```python
from build123d import *

# Parameters (mm, degrees)
SKETCH_1_W          = 15
SKETCH_1_H          = 170
EXTRUDE_1_DEPTH     = 12
SKETCH_2_W          = 8.1
SKETCH_2_H          = 10.1
CUT_EXTRUDE_1_DEPTH = 20.5
CUT_EXTRUDE_2_REACH = 89.144
SKETCH_3_R          = 2.1
SKETCH_5_R          = 2.1
CUT_EXTRUDE_3_DEPTH = 12
SKETCH_6_W          = 15
SKETCH_6_H          = 12
CUT_EXTRUDE_4_DEPTH = 2


with BuildPart() as part:
    # 草图1 → 凸台-拉伸1 (new body)
    with BuildSketch(Plane.XY):
        Rectangle(SKETCH_1_W, SKETCH_1_H)
    extrude(amount=EXTRUDE_1_DEPTH)

    # 草图2 → 切除-拉伸1 (cut)
    with BuildSketch(Plane.XZ.offset(85)):
        with Locations((-1.5, 5.05)):
            Rectangle(SKETCH_2_W, SKETCH_2_H)
    extrude(amount=-CUT_EXTRUDE_1_DEPTH, mode=Mode.SUBTRACT)

    # 切除-拉伸2: up to this face of the body (flat: up to its plane)
    cut_extrude_2_end = Plane(part.part.faces().sort_by_distance((-7.5, 0, 6))[0])
    # 草图3 → 切除-拉伸2 (cut, up to the picked face)
    with BuildSketch(Plane(origin=(7.5, 0, 0), x_dir=(0, 0, -1), z_dir=(1, 0, 0)), mode=Mode.PRIVATE) as cut_extrude_2_sk1:
        with Locations((-5, -69.75)):
            Circle(SKETCH_3_R)
    cut_extrude_2_tool1 = split(extrude(cut_extrude_2_sk1.sketch, amount=-CUT_EXTRUDE_2_REACH, mode=Mode.PRIVATE), bisect_by=cut_extrude_2_end, keep=Keep.BOTH, mode=Mode.PRIVATE)
    # 草图3 → 切除-拉伸2 (cut, up to the picked face)
    with BuildSketch(Plane(origin=(7.5, 0, 0), x_dir=(0, 0, -1), z_dir=(1, 0, 0)), mode=Mode.PRIVATE) as cut_extrude_2_sk2:
        with Locations((-5, -78.75)):
            Circle(SKETCH_3_R)
    cut_extrude_2_tool2 = split(extrude(cut_extrude_2_sk2.sketch, amount=-CUT_EXTRUDE_2_REACH, mode=Mode.PRIVATE), bisect_by=cut_extrude_2_end, keep=Keep.BOTH, mode=Mode.PRIVATE)
    add(cut_extrude_2_tool1.solids().sort_by(Axis((7.5, -69.75, 5), (-1, 0, 0)))[0], mode=Mode.SUBTRACT)
    add(cut_extrude_2_tool2.solids().sort_by(Axis((7.5, -78.75, 5), (-1, 0, 0)))[0], mode=Mode.SUBTRACT)

    # 草图5 → 切除-拉伸3 (cut)
    with BuildSketch(Plane.XY.offset(12)):
        with Locations((0, -27)):
            Circle(SKETCH_5_R)
        with Locations((0, -35)):
            Circle(SKETCH_5_R)
        with Locations((0, -19)):
            Circle(SKETCH_5_R)
        with Locations((0, -11)):
            Circle(SKETCH_5_R)
        with Locations((0, -3)):
            Circle(SKETCH_5_R)
        with Locations((0, 5)):
            Circle(SKETCH_5_R)
        with Locations((0, 13)):
            Circle(SKETCH_5_R)
        with Locations((0, 21)):
            Circle(SKETCH_5_R)
        with Locations((0, 29)):
            Circle(SKETCH_5_R)
        with Locations((0, 37)):
            Circle(SKETCH_5_R)
        with Locations((0, 45)):
            Circle(SKETCH_5_R)
        with Locations((0, 53)):
            Circle(SKETCH_5_R)
        with Locations((0, 61)):
            Circle(SKETCH_5_R)
        with Locations((0, 69)):
            Circle(SKETCH_5_R)
    extrude(amount=-CUT_EXTRUDE_3_DEPTH, mode=Mode.SUBTRACT)

    # 草图6 → 切除-拉伸4 (cut)
    with BuildSketch(Plane.XZ.offset(85)):
        with Locations((0, 6)):
            Rectangle(SKETCH_6_W, SKETCH_6_H)
    extrude(amount=-CUT_EXTRUDE_4_DEPTH, mode=Mode.SUBTRACT)


solid = part.part
```
Input: part model. Units: mm. Frame: model coordinates. A direction names the side the tool comes from. Give positions to 0.01 mm unless a question says otherwise; leave off trailing zeros. Order: outer loops, then holes, each group sorted by start corner. A loop starts at its lowest first (then second) coordinate and runs counter-clockwise, first axis right, second up. Notation, with made-up numbers: M 11,55 L 63,55 A24 ccw 63,82 Z; hole C -18.75,9.25 d4. An arc over 180 degrees is marked long. Return JSON: item names as keys, results as strings.
1) Section query B-B on y = 5. Output: boundary loops of the cut face in (x, z), and give its area (3 significant figures).
Taken from the geometry:
{"outline": "M -7.5,0 L -2.1,0 L -2.1,12 L -7.5,12 Z; M 2.1,0 L 7.5,0 L 7.5,12 L 2.1,12 Z", "area": "130 mm2"}
2) Section query C-C on x = 0. Count the separate pieces of the cut face and the enclosed holes in it, and give its area (3 significant figures).
Taken from the geometry:
{"separate pieces": "15", "enclosed holes": "0", "area": "1,120 mm2"}
3) Contact query for flat-ended pins moving along their axis: pin 1 (5 mm diameter, centred on x = 0, y = 37, fed in from +Z); pin 2 (3.5 mm diameter, centred on x = 0, y = -19, fed in from +Z). Output: stop coordinate, or through.
Taken from the geometry:
{"pin 1": "stops at z = 12", "pin 2": "passes through"}
4) Mould query, pull axis Z, two halves, no side actions, for faces 1 (the face through (0, 2, 0)), 2 (the face through (0, 2, 12)), 3 (the face through (-6.511, -80.028, 6.666)), 4 (the face through (-1.666, 67.722, 6.084)). Classes: released by +Z, released by -Z, zero draft, split by the parting line, or undercut.
Taken from the geometry:
{"face 1": "released by -Z", "face 2": "released by +Z", "face 3": "undercut", "face 4": "zero draft"}
5) Access query for faces 5 (the face through (2.55, -74, 5)), 6 (the face through (0.969, 27.137, 6.084)). Directions: +Z, -Z, +X, -X, +Y, -Y. A direction counts if a zero-diameter tool reaches every point of the face in a straight line with its end or side. Return the directions, or none.
Taken from the geometry:
{"face 5": "-Z, -Y", "face 6": "+Z, -Z"}
6) Line query: L1, parallel to Y at x = 3.6, z = 5; L2, parallel to Y at x = -2.5, z = 2.75; L3, parallel to X at y = 46, z = 1.5. Output: solid intervals per line, ascending. Write a range as [from, to].
Taken from the geometry:
{"L1": "y = [-83, -80.85], [-76.65, -71.85], [-67.65, 85]", "L2": "y = [-64.5, 85]", "L3": "x = [-7.5, -1.85], [1.85, 7.5]"}
7) Section query A-A on y = -78.75. Output: boundary loops of the cut face in (x, z), and give its area (3 significant figures).
Taken from the geometry:
{"outline": "M -7.5,0 L -5.55,0 L -5.55,2.9 L -7.5,2.9 Z; M -7.5,7.1 L -5.55,7.1 L -5.55,10.1 L 2.55,10.1 L 2.55,7.1 L 7.5,7.1 L 7.5,12 L -7.5,12 Z; M 2.55,0 L 7.5,0 L 7.5,2.9 L 2.55,2.9 Z", "area": "69.2 mm2"}
